```python
from build123d import *

# Parameters (mm, degrees)
SKETCH_1_W                   = 66
SKETCH_1_H                   = 30
EXTRUDE_1_DEPTH              = 18.5
SKETCH_2_R                   = 25
CUT_EXTRUDE_1_DEPTH          = 75.821454143
HOLE_WIZARD_M4_1_D           = 4.8
HOLE_WIZARD_M4_1_CBORE_D     = 8
HOLE_WIZARD_M4_1_CBORE_DEPTH = 4


with BuildPart() as part:
    # 草图1 → 凸台-拉伸1 (new body)
    with BuildSketch(Plane.XY):
        with Locations((33, 15)):
            Rectangle(SKETCH_1_W, SKETCH_1_H)
    extrude(amount=EXTRUDE_1_DEPTH)

    # 草图2 → 切除-拉伸1 (cut, through all)
    with BuildSketch(Plane.XY.offset(18.5)):
        with Locations((33, 30)):
            Circle(SKETCH_2_R)
    extrude(amount=-CUT_EXTRUDE_1_DEPTH, mode=Mode.SUBTRACT)

    # M4 六角凹头螺钉的柱形沉头孔1 (through all)
    with Locations(Plane.XZ):
        with Locations((5, 13.75), (5, 4.75), (61, 13.75), (61, 4.75)):
            CounterBoreHole(HOLE_WIZARD_M4_1_D / 2, HOLE_WIZARD_M4_1_CBORE_D / 2, HOLE_WIZARD_M4_1_CBORE_DEPTH)


solid = part.part
```
For this review, take the finished solid that the model builds, in its own axes (mm). A direction names the side the tool comes from. Give positions to 0.01 mm unless a question says otherwise; leave off trailing zeros. Write each loop counter-clockwise with the first axis right and the second up, starting at its lowest first coordinate (ties: lowest second). Pieces come first, ordered by that corner, then holes. Notation, with made-up numbers: M 19.25,24.5 L 23.25,24.5 A24 ccw 23.25,57.5 Z; hole C 25,-17 d5. An arc over 180 degrees is marked long. Answer as CSV lines item,"result".
1. For faces 1 (the flat face through (0, 15, 9)), 2 (the cylindrical face through (4.133, 1.972, 0.845)), list the 3-axis set-ups (+Z, -Z, +X, -X, +Y, -Y) from which the entire face can be reached by the end or side of a thin tool; tool diameter is ignored.
Findings:
face 1,"+Z, -Z, -X, +Y, -Y"
face 2,"-Y"
2. For pin 1 (5 mm diameter, centred on x = 5, z = 13.75, fed in from -Y); pin 2 (2 mm diameter, centred on x = 11.5, z = 8, fed in from +Y); pin 3 (1.5 mm diameter, centred on x = 14.5, z = 10.5, fed in from +Y), all flat-tipped, find the tip position at first contact; note any pin that passes through.
Findings:
pin 1,"stops at y = 4"
pin 2,"stops at y = 19.1"
pin 3,"stops at y = 14.05"
3. Consider section A-A, the plane z = 13.75. Write out the cut boundary in (x, y).
Findings:
outline,"M 0,0 L 1,0 L 1,4 L 2.6,4 L 2.6,30 L 0,30 Z; M 7.4,4 L 9,4 L 9,0 L 57,0 L 57,4 L 58.6,4 L 58.6,30 L 58,30 A25 cw 8,30 L 7.4,30 Z; M 63.4,4 L 65,4 L 65,0 L 66,0 L 66,30 L 63.4,30 Z"
4. Consider section D-D, the plane y = 25. Write out the cut boundary in (x, z), then the cut area to 3 significant figures.
Findings:
outline,"M 0,0 L 8.51,0 L 8.51,18.5 L 0,18.5 Z; M 57.49,0 L 66,0 L 66,18.5 L 57.49,18.5 Z; hole C 5,4.75 d4.8; hole C 5,13.75 d4.8; hole C 61,4.75 d4.8; hole C 61,13.75 d4.8"
area,"242 mm2"
5. Wall thickness on line 1 (Z direction, x = 61, y = 1); line 2 (Z direction, x = 61, y = 22.75); line 3 (X direction, y = 11.5, z = 2.75): over which ranges is each line inside the solid? List them lowest first.
Findings:
line 1,"z = 0 to 0.75, 8.75 to 9.75, 17.75 to 18.5"
line 2,"z = 0 to 2.35, 7.15 to 11.35, 16.15 to 18.5"
line 3,"x = 0 to 3.67, 6.33 to 16.18, 49.82 to 59.67, 62.33 to 66"
6. Consider section C-C, the plane x = 5. Write out the cut boundary in (y, z).
Findings:
outline,"M 0,0 L 30,0 L 30,2.35 L 4,2.35 L 4,0.75 L 0,0.75 Z; M 0,8.75 L 4,8.75 L 4,7.15 L 30,7.15 L 30,11.35 L 4,11.35 L 4,9.75 L 0,9.75 Z; M 0,17.75 L 4,17.75 L 4,16.15 L 30,16.15 L 30,18.5 L 0,18.5 Z"
7. Draft analysis for pull direction Z (two halves, no side actions). For faces 3 (the flat face through (7, 4, 12)), 4 (the flat face through (33, 0, 9)), 5 (the cylindrical face through (3.71, 17.182, 6.774)), 6 (the flat face through (25, 5, 18.5)), state which applies: +Z half, -Z half, draft (parallel to the pull), parting line (faces both ways), or undercut.
Findings:
face 3,"undercut"
face 4,"draft"
face 5,"undercut"
face 6,"+Z half"
8. Consider section B-B, the plane y = 7. Write out the cut boundary in (x, z), then the cut area to 3 significant figures.
Findings:
outline,"M 0,0 L 23.2,0 L 23.2,18.5 L 0,18.5 Z; M 42.8,0 L 66,0 L 66,18.5 L 42.8,18.5 Z; hole C 5,4.75 d4.8; hole C 5,13.75 d4.8; hole C 61,4.75 d4.8; hole C 61,13.75 d4.8"
area,"786 mm2"
